Verification items for the finished model (mm, model axes). Round coordinates to 2 decimals unless told otherwise and drop trailing zeros. Write each loop counter-clockwise with the first axis right and the second up, starting at its lowest first coordinate (ties: lowest second). Pieces come first, ordered by that corner, then holes. Notation, with made-up numbers: M 63,58 L 68,58 A20 ccw 68,96 Z; hole C 23,76.25 d11. An arc over 180 degrees is marked long. Write each question's results on one line, items separated by ' | '.
Autodesk Inventor part; units mm, degrees
ref_plane "Work Plane1" through (0, 0, 0) normal (0, 0, 1) x (1, 0, 0)
ref_plane "YZ Plane" through (0, 0, 0) normal (1, 0, 0) x (0, 1, 0)
ref_plane "XZ Plane" through (0, 0, 0) normal (0, 1, 0) x (-1, 0, 0)
ref_plane "Work Plane1" through (0, 0, 0) normal (0, 0, 1) x (1, 0, 0)
sketch "Sketch1" plane through (0, 0, 0) normal (0, 0, 1) x (1, 0, 0)
  circle A0 centre (31.2751, 14.3567) radius 2.032
  circle A1 centre (-31.2751, -10.7579) radius 2.032
  circle A2 centre (-9.1964, -21.5433) radius 2.032
  line L0 (4.4799, 27.3609) -> (32.7659, 20.5292)
  arc A3 (4.4799, 27.3609) -> (-15.0435, 20.5211) centre (0.0075, 8.8433) ccw
  line L1 (-36.2921, -6.8653) -> (-15.0435, 20.5211)
  arc A4 (-36.2921, -6.8653) -> (-27.8312, -16.0929) centre (-31.2751, -10.7579) ccw
  arc A5 (-19.0523, -17.9839) -> (-27.8312, -16.0929) centre (-24.3873, -21.4279) ccw
  line L2 (-14.5314, -24.9873) -> (-19.0523, -17.9839)
  arc A6 (36.9334, 11.4747) -> (32.7659, 20.5292) centre (31.2751, 14.3567) ccw
  arc A7 (-14.5314, -24.9873) -> (-5.9915, -27.0252) centre (-9.1964, -21.5433) ccw
  arc A8 (25.6029, -8.5539) -> (28.0563, -5.954) centre (22.398, -3.072) ccw
  circle A9 centre (22.398, -3.072) radius 2.032 construction
  line L3 (36.9334, 11.4747) -> (28.0563, -5.954)
  line L4 (25.6029, -8.5539) -> (-5.9915, -27.0252)
  line L5 (72.5061, 7.5054) -> (72.5061, 11.8054)
  circle A10 centre (0.0075, 8.8433) radius 2.2225
  point P0 (0, 0)
  dimension "d14" = 4.064
  dimension "d16" = 4.445
extrude "Plate3" add sketch "Sketch1" along normal blind 1.5875 contours L0 A6 L3 A8 L4 A7 L2 A5 A4 L1 A3 | A10
sketch "Sketch2" plane through (0, 0, 1.5875) normal (0, 0, 1) x (1, 0, 0)
  arc A0 (-36.2921, -6.8653) -> (-27.8312, -16.0929) centre (-31.2751, -10.7579) ccw
  circle A1 centre (-31.2751, -10.7579) radius 2.032
  line L0 (-36.2921, -6.8653) -> (-15.0435, 20.5211)
  arc A2 (4.4799, 27.3609) -> (-15.0435, 20.5211) centre (0.0075, 8.8433) ccw
  line L1 (4.4799, 27.3609) -> (32.7659, 20.5292)
  arc A3 (36.9334, 11.4747) -> (32.7659, 20.5292) centre (31.2751, 14.3567) ccw
  circle A4 centre (31.2751, 14.3567) radius 2.032
  line L2 (36.9334, 11.4747) -> (28.0563, -5.954)
  arc A5 (25.6029, -8.5539) -> (28.0563, -5.954) centre (22.398, -3.072) ccw
  line L3 (25.6029, -8.5539) -> (-5.9915, -27.0252)
  arc A6 (-14.5314, -24.9873) -> (-5.9915, -27.0252) centre (-9.1964, -21.5433) ccw
  line L4 (-14.5314, -24.9873) -> (-19.0523, -17.9839)
  arc A7 (-19.0523, -17.9839) -> (-27.8312, -16.0929) centre (-24.3873, -21.4279) ccw
  circle A8 centre (-9.1964, -21.5433) radius 2.032
  circle A9 centre (0.0075, 8.8433) radius 2.2225
  point P0 (0, 0)
  dimension "d17" = 4.445
extrude "Extrusion1" cut sketch "Sketch2" against normal blind 38.1 contours A9
equation "\"d15\" = Thickness"
equation "\"BendRadius\" = Thickness"
equation "\"BendReliefWidth\" = Thickness"
equation "\"BendReliefDepth\" = 0.5 * Thickness"
equation "\"CornerReliefSize\" = 4 * Thickness"
equation "\"MinimumRemnant\" = 2 * Thickness"
equation "\"TransitionRadius\" = BendRadius"
equation "\"JacobiRadiusSize\" = BendRadius"
equation "\"GapSize\" = Thickness"
properties part number "Front Horizontal Odom Pod Rot Side" material "Acetal Resin, White"
1) Sectioned sample at B-B, the plane z = 0.65. Record the cut outline in (x, y) (1 decimal), and give its area (3 significant figures).
Calculated:
outline: M -36.3,-6.9 A6.4 ccw -27.8,-16.1 A6.3 cw -19.1,-18 L -14.5,-25 A6.3 ccw -6,-27 L 25.6,-8.6 A6.3 ccw 28.1,-6 L 36.9,11.5 A6.3 ccw 32.8,20.5 L 4.5,27.4 A19.1 ccw -15,20.5 Z; hole C -31.3,-10.8 d4.1; hole C -9.2,-21.5 d4.1; hole C 0,8.8 d4.4; hole C 31.3,14.4 d4.1 | area: 2,530 mm²
2) Sectioned sample at D-D, the plane x = 10.5. Record the cut outline in (y, z).
Calculated:
outline: M -17.38,0 L 25.91,0 L 25.91,1.59 L -17.38,1.59 Z
3) Sectioned sample at A-A, the plane x = -0.5. Record the cut outline in (y, z).
Calculated:
outline: M -23.81,0 L 6.68,0 L 6.68,1.59 L -23.81,1.59 Z; M 11.01,0 L 27.89,0 L 27.89,1.59 L 11.01,1.59 Z
4) Sectioned sample at C-C, the plane y = 23. Record the cut outline in (x, z), and give its area (3 significant figures).
Calculated:
outline: M -12.74,0 L 22.54,0 L 22.54,1.59 L -12.74,1.59 Z | area: 56.0 mm²
5) Material ranges on line 1 (X direction, y = 13, z = 0.9); line 2 (X direction, y = -21, z = 0.85); line 3 (Y direction, x = 30.5, z = 1.1), recorded low to high. Write a range as [from, to].
Calculated:
line 1: x = [-20.88, 29.76], [32.79, 37.48] | line 2: x = [-17.11, -11.15], [-7.24, 4.31] | line 3: y = [-1.16, 12.48], [16.24, 21.08]
6) Depth check by flat-ended pin: P1, Ø3.5, axis at x = 31.28, y = 14.36, coming from the -Z side. Enter the tip coordinate at first touch or a pass-through.
Calculated:
P1: passes through
